Check sheet for the modelled part. Datum: model origin and axes. Units: mm. A direction names the side the tool comes from. Round coordinates to 2 decimals unless told otherwise and drop trailing zeros. Write each loop counter-clockwise with the first axis right and the second up, starting at its lowest first coordinate (ties: lowest second). Pieces come first, ordered by that corner, then holes. Notation, with made-up numbers: M 39.5,43 L 54.5,43 A29 cw 54.5,65 Z; hole C -3,74.25 d5. An arc over 180 degrees is marked long. One line per item, written item: value.
from build123d import *

# Parameters (mm, degrees)
SKETCH1_W                    = 736.6
SKETCH1_H                    = 736.6
BOSS_EXTRUDE1_DEPTH          = 50.8
SHELL1_T                     = -1.5875
CONVERT_SOLID1_START         = -368.3
CONVERT_SOLID1_DEPTH         = 4.587500016
CONVERT_SOLID1_START_2       = 363.712499984
CONVERT_SOLID1_2_DEPTH       = 4.587500016
CONVERT_SOLID1_START_3       = -363.712499984
CONVERT_SOLID1_3_DEPTH       = 727.424999968
CONVERT_SOLID1_START_4       = -376.7125
CONVERT_SOLID1_4_DEPTH       = 10.500000016
CONVERT_SOLID1_START_5       = 366.212499984
CONVERT_SOLID1_5_DEPTH       = 10.500000016
CONVERT_SOLID1_START_6       = -371.7125
CONVERT_SOLID1_6_OUTLINE_W   = 727.424999968
CONVERT_SOLID1_6_OUTLINE_H   = 8.4125
CONVERT_SOLID1_6_OUTLINE_W_2 = 10
CONVERT_SOLID1_6_OUTLINE_H_2 = 46.212499984
CONVERT_SOLID1_6_DEPTH       = 743.425
CONVERT_SOLID1_START_7       = -366.2125
CONVERT_SOLID1_7_DEPTH       = 732.425
CONVERT_SOLID1_START_8       = -366.7125
CONVERT_SOLID1_8_OUTLINE_W   = 49.2125
CONVERT_SOLID1_8_OUTLINE_H   = 1.5875
CONVERT_SOLID1_8_DEPTH       = 0.5
CONVERT_SOLID1_START_9       = 366.2125
CONVERT_SOLID1_9_OUTLINE_W   = 49.2125
CONVERT_SOLID1_9_OUTLINE_H   = 1.5875
CONVERT_SOLID1_9_DEPTH       = 0.5
CONVERT_SOLID1_10_OUTLINE_W  = 3.000000016
CONVERT_SOLID1_10_OUTLINE_H  = 1.5875
CONVERT_SOLID1_10_DEPTH      = 2.500000016
CONVERT_SOLID1_11_OUTLINE_W  = 3.000000016
CONVERT_SOLID1_11_OUTLINE_H  = 1.5875
CONVERT_SOLID1_11_DEPTH      = 2.500000016


with BuildPart() as part:
    # Sketch1 → Boss-Extrude1 (new body)
    with BuildSketch(Plane(origin=(0, 0, 0), x_dir=(1, 0, 0), z_dir=(0, 1, 0))):
        Rectangle(SKETCH1_W, SKETCH1_H)
    extrude(amount=BOSS_EXTRUDE1_DEPTH)

    # Shell1
    shell1_openings = [part.faces().sort_by_distance(p)[0] for p in [
        (0, 50.8, 0),
    ]]
    offset(amount=SHELL1_T, openings=shell1_openings, kind=Kind.INTERSECTION)

    # Convert-Solid1: read off the stored shape, not the designer's step
    # Convert-Solid1 outline → Convert-Solid1 (cut)
    with BuildSketch(Plane.XY.offset(CONVERT_SOLID1_START)):
        with BuildLine():
            Line((366.212499984, 1.5875), (363.712499984, 1.5875))
            Line((363.712499984, 1.5875), (363.712499984, 0))
            Line((363.712499984, 0), (368.3, 0))
            Line((368.3, 0), (368.3, 4.587500016))
            Line((368.3, 4.587500016), (366.7125, 4.587500016))
            Line((366.7125, 4.587500016), (366.7125, 2.087500016))
            ThreePointArc((366.7125, 2.087500016), (366.566053386, 1.733946614), (366.212499984, 1.5875))
        make_face()
        with BuildLine():
            Line((-363.712499984, 0), (-363.712499984, 1.5875))
            Line((-363.712499984, 1.5875), (-366.212499984, 1.5875))
            ThreePointArc((-366.212499984, 1.5875), (-366.566053386, 1.733946614), (-366.7125, 2.087500016))
            Line((-366.7125, 2.087500016), (-366.7125, 4.587500016))
            Line((-366.7125, 4.587500016), (-368.3, 4.587500016))
            Line((-368.3, 4.587500016), (-368.3, 0))
            Line((-368.3, 0), (-363.712499984, 0))
        make_face()
    extrude(amount=CONVERT_SOLID1_DEPTH, mode=Mode.SUBTRACT)

    # Convert-Solid1 2 outline → Convert-Solid1 2 (cut)
    with BuildSketch(Plane.XY.offset(CONVERT_SOLID1_START_2)):
        with BuildLine():
            Line((366.212499984, 1.5875), (363.712499984, 1.5875))
            Line((363.712499984, 1.5875), (363.712499984, 0))
            Line((363.712499984, 0), (368.3, 0))
            Line((368.3, 0), (368.3, 4.587500016))
            Line((368.3, 4.587500016), (366.7125, 4.587500016))
            Line((366.7125, 4.587500016), (366.7125, 2.087500016))
            ThreePointArc((366.7125, 2.087500016), (366.566053386, 1.733946614), (366.212499984, 1.5875))
        make_face()
        with BuildLine():
            Line((-363.712499984, 0), (-363.712499984, 1.5875))
            Line((-363.712499984, 1.5875), (-366.212499984, 1.5875))
            ThreePointArc((-366.212499984, 1.5875), (-366.566053386, 1.733946614), (-366.7125, 2.087500016))
            Line((-366.7125, 2.087500016), (-366.7125, 4.587500016))
            Line((-366.7125, 4.587500016), (-368.3, 4.587500016))
            Line((-368.3, 4.587500016), (-368.3, 0))
            Line((-368.3, 0), (-363.712499984, 0))
        make_face()
    extrude(amount=CONVERT_SOLID1_2_DEPTH, mode=Mode.SUBTRACT)

    # Convert-Solid1 3 outline → Convert-Solid1 3 (add)
    with BuildSketch(Plane.XY.offset(CONVERT_SOLID1_START_3)):
        with BuildLine():
            Line((368.3, 0), (-368.3, 0))
            Line((-368.3, 0), (-368.3, 50.8))
            Line((-368.3, 50.8), (-376.7125, 50.8))
            Line((-376.7125, 50.8), (-376.7125, 2.087500016))
            ThreePointArc((-376.7125, 2.087500016), (-373.637121198, -5.337121198), (-366.212499984, -8.4125))
            Line((-366.212499984, -8.4125), (366.212499984, -8.4125))
            ThreePointArc((366.212499984, -8.4125), (373.637121198, -5.337121198), (376.7125, 2.087500016))
            Line((376.7125, 2.087500016), (376.7125, 50.8))
            Line((376.7125, 50.8), (368.3, 50.8))
            Line((368.3, 50.8), (368.3, 0))
        make_face()
        with BuildLine():
            ThreePointArc((366.7125, 2.087500016), (366.566053386, 1.733946614), (366.212499984, 1.5875))
            Line((366.212499984, 1.5875), (366.7125, 1.5875))
            Line((366.7125, 1.5875), (366.7125, 2.087500016))
        make_face()
        with BuildLine():
            Line((-366.7125, 1.5875), (-366.212499984, 1.5875))
            ThreePointArc((-366.212499984, 1.5875), (-366.566053386, 1.733946614), (-366.7125, 2.087500016))
            Line((-366.7125, 2.087500016), (-366.7125, 1.5875))
        make_face()
    extrude(amount=CONVERT_SOLID1_3_DEPTH)

    # Convert-Solid1 4 outline → Convert-Solid1 4 (add)
    with BuildSketch(Plane.XY.offset(CONVERT_SOLID1_START_4)):
        Polygon((-363.712499984, -8.4125), (363.712499984, -8.4125), (363.712499984, 4.587500016), (366.2125, 4.587500016), (366.2125, 50.8), (-366.2125, 50.8), (-366.2125, 4.587500016), (-363.712499984, 4.587500016), align=None)
    extrude(amount=CONVERT_SOLID1_4_DEPTH)

    # Convert-Solid1 5 outline → Convert-Solid1 5 (add)
    with BuildSketch(Plane.XY.offset(CONVERT_SOLID1_START_5)):
        Polygon((-363.712499984, -8.4125), (363.712499984, -8.4125), (363.712499984, 4.587500016), (366.2125, 4.587500016), (366.2125, 50.8), (-366.2125, 50.8), (-366.2125, 4.587500016), (-363.712499984, 4.587500016), align=None)
    extrude(amount=CONVERT_SOLID1_5_DEPTH)

    # Convert-Solid1 6 outline → Convert-Solid1 6 (add)
    with BuildSketch(Plane.XY.offset(CONVERT_SOLID1_START_6)):
        with Locations((0, -4.20625)):
            Rectangle(CONVERT_SOLID1_6_OUTLINE_W, CONVERT_SOLID1_6_OUTLINE_H)
        with Locations((371.7125, 27.693750008)):
            Rectangle(CONVERT_SOLID1_6_OUTLINE_W_2, CONVERT_SOLID1_6_OUTLINE_H_2)
        with Locations((-371.7125, 27.693750008)):
            Rectangle(CONVERT_SOLID1_6_OUTLINE_W_2, CONVERT_SOLID1_6_OUTLINE_H_2)
    extrude(amount=CONVERT_SOLID1_6_DEPTH)

    # Convert-Solid1 7 outline → Convert-Solid1 7 (cut)
    with BuildSketch(Plane.YZ.offset(CONVERT_SOLID1_START_7)):
        with BuildLine():
            Line((50.8, -366.212499984), (1.5875, -366.212499984))
            ThreePointArc((1.5875, -366.212499984), (1.733946614, -366.566053386), (2.087500016, -366.7125))
            Line((2.087500016, -366.7125), (50.8, -366.7125))
            Line((50.8, -366.7125), (50.8, -366.212499984))
        make_face()
        with BuildLine():
            Line((50.8, 366.212499984), (50.8, 366.7125))
            Line((50.8, 366.7125), (2.087500016, 366.7125))
            ThreePointArc((2.087500016, 366.7125), (1.733946614, 366.566053386), (1.5875, 366.212499984))
            Line((1.5875, 366.212499984), (50.8, 366.212499984))
        make_face()
        with BuildLine():
            Line((-8.4125, -376.7125), (2.087500016, -376.7125))
            ThreePointArc((2.087500016, -376.7125), (-5.337121198, -373.637121198), (-8.4125, -366.212499984))
            Line((-8.4125, -366.212499984), (-8.4125, -376.7125))
        make_face()
        with BuildLine():
            Line((-8.4125, 376.7125), (-8.4125, 366.212499984))
            ThreePointArc((-8.4125, 366.212499984), (-5.337121198, 373.637121198), (2.087500016, 376.7125))
            Line((2.087500016, 376.7125), (-8.4125, 376.7125))
        make_face()
    extrude(amount=CONVERT_SOLID1_7_DEPTH, mode=Mode.SUBTRACT)

    # Convert-Solid1 8 outline → Convert-Solid1 8 (cut)
    with BuildSketch(Plane.YZ.offset(CONVERT_SOLID1_START_8)):
        with Locations((26.19375, -367.50625)):
            Rectangle(CONVERT_SOLID1_8_OUTLINE_W, CONVERT_SOLID1_8_OUTLINE_H)
        with Locations((26.19375, 367.50625)):
            Rectangle(CONVERT_SOLID1_8_OUTLINE_W, CONVERT_SOLID1_8_OUTLINE_H)
    extrude(amount=CONVERT_SOLID1_8_DEPTH, mode=Mode.SUBTRACT)

    # Convert-Solid1 9 outline → Convert-Solid1 9 (cut)
    with BuildSketch(Plane.YZ.offset(CONVERT_SOLID1_START_9)):
        with Locations((26.19375, -367.50625)):
            Rectangle(CONVERT_SOLID1_9_OUTLINE_W, CONVERT_SOLID1_9_OUTLINE_H)
        with Locations((26.19375, 367.50625)):
            Rectangle(CONVERT_SOLID1_9_OUTLINE_W, CONVERT_SOLID1_9_OUTLINE_H)
    extrude(amount=CONVERT_SOLID1_9_DEPTH, mode=Mode.SUBTRACT)

    # Convert-Solid1 10 outline → Convert-Solid1 10 (cut)
    with BuildSketch(Plane.YZ.offset(CONVERT_SOLID1_START_7)):
        with Locations((3.087500008, -367.50625)):
            Rectangle(CONVERT_SOLID1_10_OUTLINE_W, CONVERT_SOLID1_10_OUTLINE_H)
        with Locations((3.087500008, 367.50625)):
            Rectangle(CONVERT_SOLID1_10_OUTLINE_W, CONVERT_SOLID1_10_OUTLINE_H)
    extrude(amount=CONVERT_SOLID1_10_DEPTH, mode=Mode.SUBTRACT)

    # Convert-Solid1 11 outline → Convert-Solid1 11 (cut)
    with BuildSketch(Plane.YZ.offset(CONVERT_SOLID1_START_2)):
        with Locations((3.087500008, -367.50625)):
            Rectangle(CONVERT_SOLID1_11_OUTLINE_W, CONVERT_SOLID1_11_OUTLINE_H)
        with Locations((3.087500008, 367.50625)):
            Rectangle(CONVERT_SOLID1_11_OUTLINE_W, CONVERT_SOLID1_11_OUTLINE_H)
    extrude(amount=CONVERT_SOLID1_11_DEPTH, mode=Mode.SUBTRACT)


solid = part.part
Q1. Depth check by flat-ended pin: P1, Ø6, axis at x = 157, z = 196, coming from the +Y side; P2, Ø6.5, axis at x = 373, y = -3, coming from the +Z side; P3, Ø0.8, axis at x = 364.5, z = -374, coming from the -Y side. Enter the tip coordinate at first touch or a pass-through.
Completed:
P1: y = 1.59
P2: z = 363.71
P3: y = 4.59
Q2. Scan lines: line 1 (Z direction, x = 15, y = 6); line 2 (Y direction, x = -49, z = 179.5). Record each from-to range of solid material in increasing order. Write a range as [from, to].
Completed:
line 1: [-376.71, -366.71], [366.71, 376.71]
line 2: [-8.41, 1.59]
Q3. Access from +Z, -Z, +X, -X, +Y, -Y to the whole of each face (thin tool, end or side, straight path). Record for faces 4 (the flat face through (-5, 26, -366.713)), 5 (the flat face through (-5, -8.412, -5)).
Completed:
face 4: +Y
face 5: +Z, -Z, +X, -X, -Y
Q4. Sectioned sample at A-A on y = 17. Enter the section's corners in (x, z), and give its area (3 significant figures).
Completed:
outline: M -376.71,-371.71 L -366.71,-371.71 L -366.71,371.71 L -376.71,371.71 Z; M -366.21,-376.71 L 366.21,-376.71 L 366.21,-366.71 L -366.21,-366.71 Z; M -366.21,366.71 L 366.21,366.71 L 366.21,376.71 L -366.21,376.71 Z; M 366.71,-371.71 L 376.71,-371.71 L 376.71,371.71 L 366.71,371.71 Z
area: 29,500 mm^2
Q5. Sectioned sample at C-C on z = 65. Enter the section's corners in (x, y).
Completed:
outline: M -376.71,2.09 A10.5 ccw -366.21,-8.41 L 366.21,-8.41 A10.5 ccw 376.71,2.09 L 376.71,50.8 L 366.71,50.8 L 366.71,2.09 A0.5 cw 366.21,1.59 L -366.21,1.59 A0.5 cw -366.71,2.09 L -366.71,50.8 L -376.71,50.8 Z
Q6. Sectioned sample at B-B on x = 100.5. Enter the section's corners in (y, z).
Completed:
outline: M -8.41,-366.21 A10.5 ccw 2.09,-376.71 L 50.8,-376.71 L 50.8,-366.71 L 2.09,-366.71 A0.5 cw 1.59,-366.21 L 1.59,366.21 A0.5 cw 2.09,366.71 L 50.8,366.71 L 50.8,376.71 L 2.09,376.71 A10.5 ccw -8.41,366.21 Z
Q7. Draft check along X on faces 1 (the flat face through (-376.712, 27, -5)), 2 (the flat face through (-5, 26, 366.713)), 3 (the flat face through (376.712, 26, -5)). Enter one of: pulls with the +X half, pulls with the -X half, needs draft (parallel to the pull), parting line crosses it, or undercut.
Completed:
face 1: pulls with the -X half
face 2: undercut
face 3: pulls with the +X half
